Input: part model. Units: mm. Frame: model coordinates. Face numbers are marked on the shaded views. A direction names the side the tool comes from. Give positions to 0.01 mm unless a question says otherwise; leave off trailing zeros. Order: outer loops, then holes, each group sorted by start corner. A loop starts at its lowest first (then second) coordinate and runs counter-clockwise, first axis right, second up.
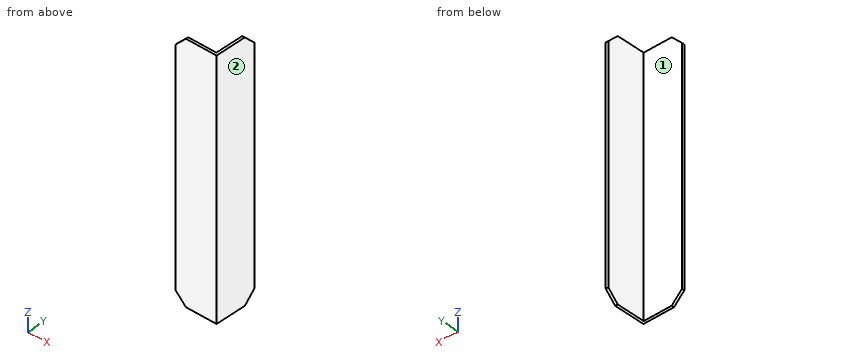
```python
from build123d import *

# Parameters (mm, degrees)
F1_DEPTH   = 609.6
F3_DEPTH   = 25.4
F1_FACE2_W = 6.35
F1_FACE2_H = 609.6
F5_DEPTH   = 25.4
F7_DEPTH   = 25.4
F9_DEPTH   = 25.4


with BuildPart() as f1:
    # F0 (on Top) → F1 (new body)
    with BuildSketch(Plane.XY):
        Polygon((21.206026165, -27.4921420044), (21.206026165, -33.8421420044), (122.6945791882, -38.5996208804), (127.4520580641, 62.8889321428), (121.1090235002, 63.1862745726), (116.5493069378, -31.9615489545), align=None)
    extrude(amount=F1_DEPTH)

    # F2 (on face) → F3 (cut)
    with BuildSketch(Plane(origin=(124.2310217623, -5.8235775776, 0), x_dir=(0.0468255795, 0.9989030809, 0), z_dir=(0.9989030809, -0.0468255795, 0))):
        Polygon((43.3879645501, 609.6), (68.7879645501, 584.2), (68.7879645501, 609.6), align=None)
    extrude(amount=-F3_DEPTH, mode=Mode.SUBTRACT)

    # F4 (on face) + F1_face2 (on face) → F5 (cut)
    with BuildSketch(Plane(origin=(-1.5364425741, -32.7760433027, 0), x_dir=(0.9989030809, -0.0468255795, 0), z_dir=(-0.0468255795, -0.9989030809, 0))):
        Polygon((22.7674427811, 584.2), (48.1674427811, 609.6), (22.7674427811, 609.6), align=None)
    with BuildSketch(Plane(origin=(21.206026165, -30.6671420044, 304.8), x_dir=(0, -1, 0), z_dir=(-1, 0, 0))):
        Rectangle(F1_FACE2_W, F1_FACE2_H)
    extrude(amount=-F5_DEPTH, dir=(-0.0468255795, -0.9989030809, 0), mode=Mode.SUBTRACT)

    # F6 (on face) → F7 (cut)
    with BuildSketch(Plane(origin=(-1.5364425741, -32.7760433027, 0), x_dir=(0.9989030809, -0.0468255795, 0), z_dir=(-0.0468255795, -0.9989030809, 0))):
        Polygon((48.1674427811, 0), (22.7674427811, 25.4), (22.7674427811, 0), align=None)
    extrude(amount=-F7_DEPTH, mode=Mode.SUBTRACT)

    # F8 (on face) → F9 (cut)
    with BuildSketch(Plane(origin=(124.2310217623, -5.8235775776, 0), x_dir=(0.0468255795, 0.9989030809, 0), z_dir=(0.9989030809, -0.0468255795, 0))):
        Polygon((68.7879645501, 25.4), (43.3879645501, 0), (68.7879645501, 0), align=None)
    extrude(amount=-F9_DEPTH, mode=Mode.SUBTRACT)


solid = f1.part
```
1) Cut plane C-C (x = 40.5). Return the cut outline in (y, z).
2) First-contact query: P1, Ø4, axis at x = 106, z = 250, coming from the +Y side; P2, Ø1, axis at y = 23.5, z = 501, coming from the -X side; P3, Ø3, axis at x = 92, z = 163, coming from the +Y side. Flat tips, straight axial feed; report the tip coordinate or a pass-through.
3) Cut plane B-B (y = -1). Return the cut outline in (x, z).
4) Reachability of the marked faces 1 and 2 from +Z, -Z, +X, -X, +Y, -Y: full face, straight path, thin tool, end or side. Return the list, or none.
5) Cut plane A-A (z = 198.5). Return the cut outline in (x, y).
6) Line query: probe 1 along X at (y, z) = (39, 273); probe 2 along Y at (x, z) = (105.5, 415.5); probe 3 along Y at (x, z) = (88.5, 181.5). Output: solid intervals per line, ascending.
Geometry says:
1. outline: (-34.75, 6.08) - (-28.4, 6.38) - (-28.4, 603.22) - (-34.75, 603.52) - close
2. P1: stops at y = -31.37
2. P2: stops at x = 119.18
2. P3: stops at y = -30.74
3. outline: (118.03, 0) - (124.46, 0) - (124.46, 609.6) - (118.03, 609.6) - close
4. face 1: +Z, -Z, +Y
4. face 2: +Z, -Z, +X, -Y
5. outline: (21.21, -33.84) - (122.69, -38.6) - (127.45, 62.89) - (121.11, 63.19) - (116.55, -31.96) - (21.5, -27.51) - close
6. probe 1: x = 119.95 to 126.33
6. probe 2: y = -37.79 to -31.44
6. probe 3: y = -37 to -30.65
